Source: three-view drawing plus pictorial views. Frame: mm from the lowest corner of the part. A direction names the side the tool comes from. Give positions to 0.01 mm unless a question says otherwise; leave off trailing zeros. Order: outer loops, then holes, each group sorted by start corner. A loop starts at its lowest first (then second) coordinate and runs counter-clockwise, first axis right, second up. Notation, with made-up numbers: (9, 74) - (47, 74) arc R18 ccw to (47, 92) - close; hole circle Ø2 at (3.5, -14). An arc over 180 degrees is marked (long way). Answer in a Markdown table with one row per item. Add a question column.
1. Mould query, pull axis Y, two halves, no side actions, for the marked faces 1, 2, 3 and 4. Classes: released by +Y, released by -Y, zero draft, split by the parting line, or undercut.
2. Access query for the marked faces 5, 6, 7 and 8. Directions: +Z, -Z, +X, -X, +Y, -Y. A direction counts if a zero-diameter tool reaches every point of the face in a straight line with its end or side. Return the directions, or none.
3. Section query B-B on z = 3.75. Return loops of the section in (x, y) (1 decimal).
4. Section query A-A on y = 10. Return loops of the section in (x, z).
5. Section query C-C on x = 3.7. Return loops of the section in (y, z).
6. Contact query for flat-ended pins moving along their axis: pin 1 (1.5 mm diameter, centred on x = 1, z = 13.5, fed in from +Y); pin 2 (1.5 mm diameter, centred on y = 3.5, z = 12, fed in from +X); pin 3 (0.6 mm diameter, centred on x = 4, z = 15.5, fed in from -Y); pin 4 (3 mm diameter, centred on x = 4, y = 8, fed in from -Z). Output: stop coordinate, or through.
7. Section query D-D on z = 16.5. Return loops of the section in (x, y).
8. Ray query, line 1 (Y direction, x = 4, z = 2.5); line 2 (Z direction, x = 3.35, y = 9.75); line 3 (Z direction, x = 2.8, y = 11.5). Return the intervals inside material, ascending. Write a range as [from, to].
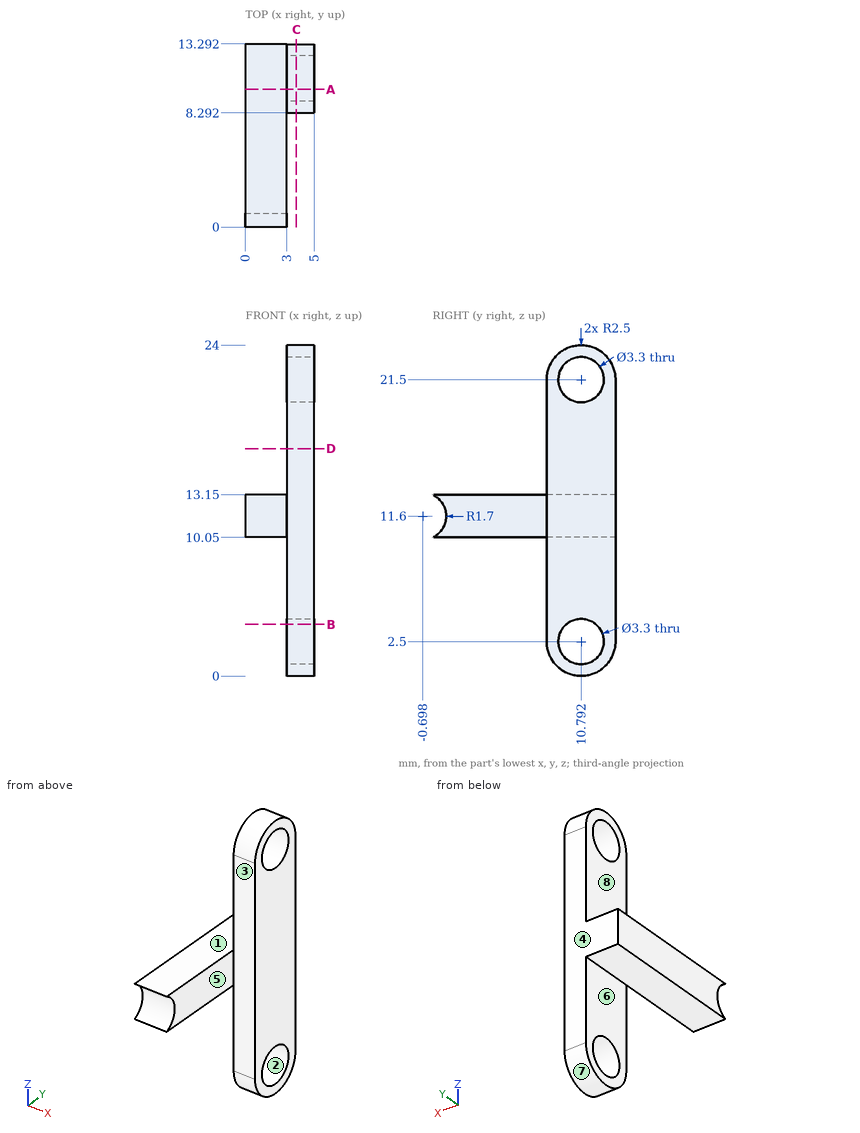
Answer:
| question | item | result |
|---|---|---|
| 1 | face 1 | zero draft |
| 1 | face 2 | undercut |
| 1 | face 3 | released by -Y |
| 1 | face 4 | released by +Y |
| 2 | face 5 | +Z, -Z, +X, -Y |
| 2 | face 6 | -Z, -X, +Y, -Y |
| 2 | face 7 | -Z, +X, -X |
| 2 | face 8 | +Z, -X, +Y, -Y |
| 3 | outline | (3, 8.3) - (5, 8.3) - (5, 9.7) - (3, 9.7) - close; (3, 11.9) - (5, 11.9) - (5, 13.3) - (3, 13.3) - close |
| 4 | outline | (0, 10.05) - (3, 10.05) - (3, 3.95) - (5, 3.95) - (5, 20.05) - (3, 20.05) - (3, 13.15) - (0, 13.15) - close; (3, 0.13) - (5, 0.13) - (5, 1.05) - (3, 1.05) - close; (3, 22.95) - (5, 22.95) - (5, 23.87) - (3, 23.87) - close |
| 5 | outline | (8.29, 2.5) arc R2.5 ccw to (13.29, 2.5) - (13.29, 21.5) arc R2.5 ccw to (8.29, 21.5) - close; hole circle Ø3.3 at (10.79, 2.5); hole circle Ø3.3 at (10.79, 21.5) |
| 6 | pin 1 | stops at y = 13.29 |
| 6 | pin 2 | stops at x = 3 |
| 6 | pin 3 | stops at y = 8.29 |
| 6 | pin 4 | stops at z = 0.36 |
| 7 | outline | (3, 8.29) - (5, 8.29) - (5, 13.29) - (3, 13.29) - close |
| 8 | line 1 | y = [8.29, 9.14], [12.44, 13.29] |
| 8 | line 2 | z = [0.23, 1.22], [3.78, 20.22], [22.78, 23.77] |
| 8 | line 3 | z = [10.05, 13.15] |
